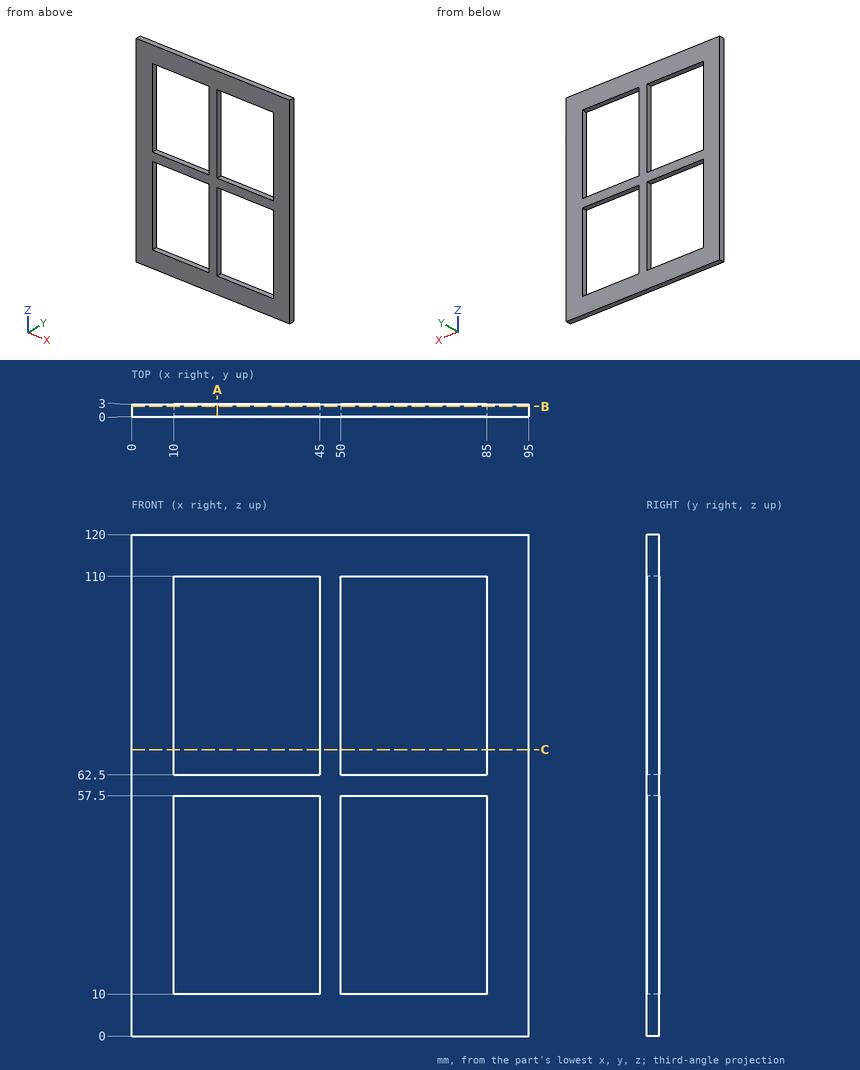
Here's the drawing with two shaded views (mm, measured from the low corner). I have some questions. Coordinates: 2 decimals unless noted, no trailing zeros. Order: outer loops, then holes, each group sorted by start corner. A loop starts at its lowest first (then second) coordinate and runs counter-clockwise, first axis right, second up. Notation, with made-up numbers: M 42,-13.75 L 89,-13.75 A5 cw 89,-5.75 Z; hole C 5,48 d1. An arc over 180 degrees is marked long. Answer as CSV lines item,"result".
Item 1: If I drill on line 1 (X direction, y = 0.95, z = 32); line 2 (Z direction, x = 11.5, y = 1), over which ranges is the centre line in solid material (lowest first)?
Results found:
line 1,"0 to 10, 45 to 50, 85 to 95"
line 2,"0 to 10, 57.5 to 62.5, 110 to 120"
Item 2: Imagine slicing it at A-A on x = 20.5. Write out the boundary of the cut face in (y, z), plus the area to 3 significant figures.
Results found:
outline,"M 0,0 L 3,0 L 3,10 L 0,10 Z; M 0,57.5 L 3,57.5 L 3,62.5 L 0,62.5 Z; M 0,110 L 3,110 L 3,120 L 0,120 Z"
area,"75.0 mm2"
Item 3: Imagine slicing it at B-B on y = 2.45. Write out the boundary of the cut face in (x, z).
Results found:
outline,"M 0,0 L 95,0 L 95,120 L 0,120 Z; hole M 10,10 L 45,10 L 45,57.5 L 10,57.5 Z; hole M 10,62.5 L 45,62.5 L 45,110 L 10,110 Z; hole M 50,10 L 85,10 L 85,57.5 L 50,57.5 Z; hole M 50,62.5 L 85,62.5 L 85,110 L 50,110 Z"
Item 4: Imagine slicing it at C-C on z = 68.5. Write out the boundary of the cut face in (x, y).
Results found:
outline,"M 0,0 L 10,0 L 10,3 L 0,3 Z; M 45,0 L 50,0 L 50,3 L 45,3 Z; M 85,0 L 95,0 L 95,3 L 85,3 Z"
